```python
from build123d import *

# Parameters (mm, degrees)
F0_W     = 1905
F0_H     = 1397
F1_DEPTH = 127
F2_W     = 765.71583
F2_H     = 142.633289
F2_W_2   = 792.600095
F2_H_2   = 142.633319
F2_H_3   = 155.145049
F2_H_4   = 150.14036
F2_H_5   = 140.555978
F2_W_3   = 768.218152
F2_H_6   = 145.560652
F2_W_4   = 765.7084
F2_H_7   = 157.647371
F2_H_8   = 160.149634
F3_DEPTH = 127.001


with BuildPart() as f1:
    # F0 (on Top) → F1 (new body)
    with BuildSketch(Plane.XY):
        with Locations((-28.528064, 26.927372)):
            Rectangle(F0_W, F0_H)
    extrude(amount=F1_DEPTH)

    # F2 (on face) → F3 (cut, through all)
    with BuildSketch(Plane.XY.offset(127)):
        with Locations((-491.099898, 548.838452)):
            Rectangle(F2_W, F2_H)
        with Locations((396.300048, 551.340818)):
            Rectangle(F2_W_2, F2_H_2)
        with Locations((-491.099898, 239.799588)):
            Rectangle(F2_W, F2_H_3)
        with Locations((396.300048, 247.306608)):
            Rectangle(F2_W_2, F2_H_4)
        with Locations((396.300048, -70.277989)):
            Rectangle(F2_W_2, F2_H_5)
        with Locations((-492.351059, -72.780326)):
            Rectangle(F2_W_3, F2_H_6)
        with Locations((-498.613023, -399.548113)):
            Rectangle(F2_W_4, F2_H_7)
        with Locations((396.300048, -400.799245)):
            Rectangle(F2_W_2, F2_H_8)
    extrude(amount=-F3_DEPTH, mode=Mode.SUBTRACT)


solid = f1.part
```
Could you check a few things on this model? Use its own coordinates, in mm. Coordinates: 2 decimals unless noted, no trailing zeros. Write each loop counter-clockwise with the first axis right and the second up, starting at its lowest first coordinate (ties: lowest second). Pieces come first, ordered by that corner, then holes. Notation, with made-up numbers: (31.25, -30.75) - (80.25, -30.75) arc R32 cw to (80.25, 3.25) - close; hole circle Ø7 at (-8.5, 29). An arc over 180 degrees is marked (long way). Use a Markdown table: item, result.
Q1. I'm going to push a flat-ended pin straight in: pin 1 Ø1 at (x, y) = (-732, -150) entering from -Z. Where does the tip first touch, or does it pass through?
Geometry check:
| item | result |
|---|---|
| pin 1 | stops at z = 0 |
Q2. Imagine slicing it at C-C (x = 190.5). List the corners of the cut face in (y, z) for me, and give its area (3 significant figures).
Geometry check:
| item | result |
|---|---|
| outline | (-671.57, 0) - (-480.87, 0) - (-480.87, 127) - (-671.57, 127) - close; (-320.72, 0) - (-140.56, 0) - (-140.56, 127) - (-320.72, 127) - close; (0, 0) - (172.24, 0) - (172.24, 127) - (0, 127) - close; (322.38, 0) - (480.02, 0) - (480.02, 127) - (322.38, 127) - close; (622.66, 0) - (725.43, 0) - (725.43, 127) - (622.66, 127) - close |
| area | 102,000 mm2 |
Q3. Imagine slicing it at A-A (y = 589.5). List the corners of the cut face in (x, z) for me.
Geometry check:
| item | result |
|---|---|
| outline | (-981.03, 0) - (-873.96, 0) - (-873.96, 127) - (-981.03, 127) - close; (-108.24, 0) - (0, 0) - (0, 127) - (-108.24, 127) - close; (792.6, 0) - (923.97, 0) - (923.97, 127) - (792.6, 127) - close |
Q4. Please list where these lines run through material, in increasing order: L1, parallel to Y at x = -215.5, z = 9; L2, parallel to X at y = -75.5, z = 45.5; L3, parallel to X at y = 265, z = 63.5.
Geometry check:
| item | result |
|---|---|
| L1 | y = -671.57 to -478.37, -320.72 to -145.56, 0 to 162.23, 317.37 to 477.52, 620.16 to 725.43 |
| L2 | x = -981.03 to -876.46, -108.24 to 0, 792.6 to 923.97 |
| L3 | x = -981.03 to -873.96, -108.24 to 0, 792.6 to 923.97 |
Q5. Thinking about a two-plate mould opening in Y: for faces 1 (the flat face through (-42, 37, 0)), 2 (the flat face through (-873.958, 548, 64)), which applies, +Y half, -Y half, draft (parallel to the pull), parting line (faces both ways), or undercut?
Geometry check:
| item | result |
|---|---|
| face 1 | draft |
| face 2 | undercut |
Q6. Imagine slicing it at B-B (x = -260). List the corners of the cut face in (y, z) for me, and give its area (3 significant figures).
Geometry check:
| item | result |
|---|---|
| outline | (-671.57, 0) - (-478.37, 0) - (-478.37, 127) - (-671.57, 127) - close; (-320.72, 0) - (-145.56, 0) - (-145.56, 127) - (-320.72, 127) - close; (0, 0) - (162.23, 0) - (162.23, 127) - (0, 127) - close; (317.37, 0) - (477.52, 0) - (477.52, 127) - (317.37, 127) - close; (620.16, 0) - (725.43, 0) - (725.43, 127) - (620.16, 127) - close |
| area | 101,000 mm2 |
Q7. Imagine slicing it at D-D (z = 54.5). Count the separate pieces of the cut face and the enclosed holes in it, and give its area (3 significant figures).
Geometry check:
| item | result |
|---|---|
| separate pieces | 1 |
| enclosed holes | 8 |
| area | 1,730,000 mm2 |
